For this review, use the dimensioned drawing (mm, ordinates from the lowest corner) and the shaded views. A direction names the side the tool comes from. Round coordinates to 2 decimals unless told otherwise and drop trailing zeros. Order: outer loops, then holes, each group sorted by start corner. A loop starts at its lowest first (then second) coordinate and runs counter-clockwise, first axis right, second up. Notation, with made-up numbers: (64, -14) - (121, -14) arc R34 ccw to (121, 21) - close; hole circle Ø3 at (-40, 89.25). An arc over 180 degrees is marked (long way). Use CSV: the item, a comma, the result in double quotes. Start each with the question number.
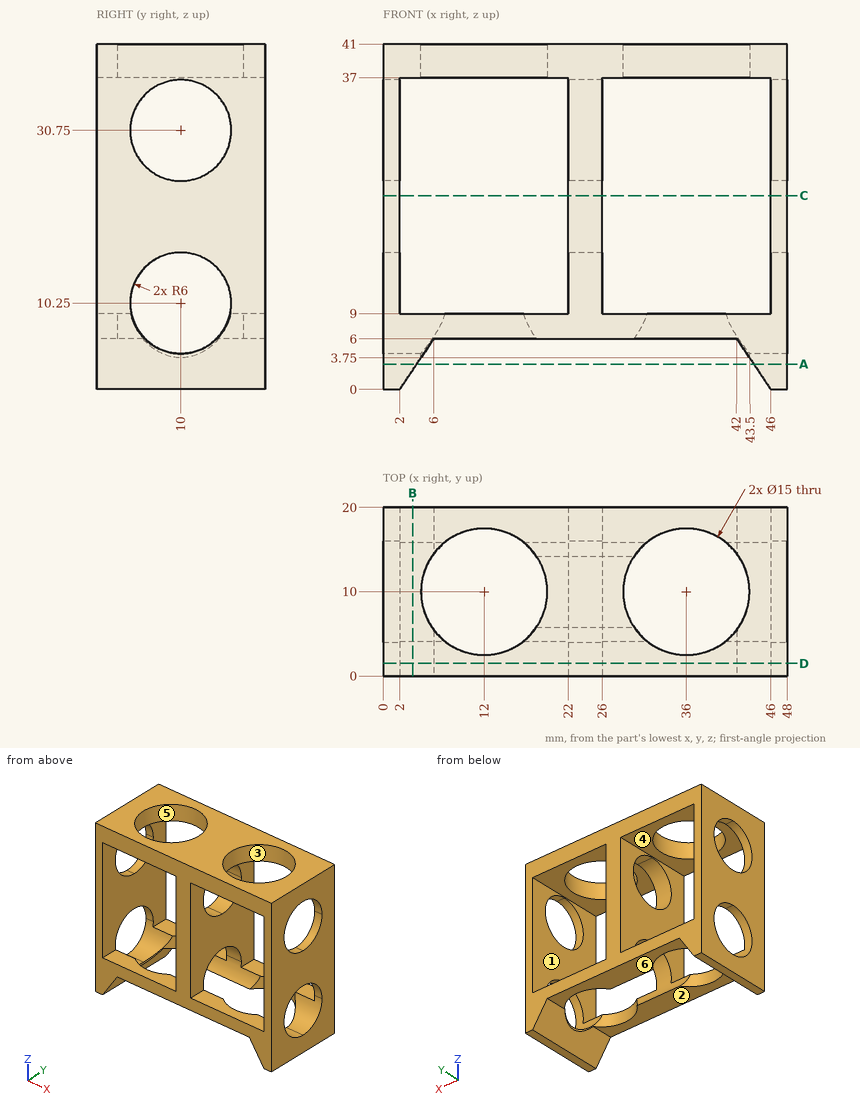
Q1. Take a section at D-D (y = 1.5). State the section outline as (x, z) points.
Q2. Take a section at B-B (x = 3.5). State the section outline as (y, z) points.
Q3. Take a section at C-C (z = 23). State the section outline as (x, y) points, plus the area to 3 significant figures.
Q4. Take a section at A-A (z = 3). State the section outline as (x, y) points, plus the area to 3 significant figures.
Q5. Clearance check with flat-ended pins moving along their axes: pin 1 (1.7 mm diameter, centred on x = 15, y = 3, fed in from -Z); pin 2 (1 mm diameter, centred on x = 25.5, y = 6.5, fed in from -Z); pin 3 (10 mm diameter, centred on x = 42, z = 25.5, fed in from -Y). State where each tip first meets the part, or that it passes through.
Q6. Tool access review of the marked faces 1, 2 and 3: name each direction out of +Z, -Z, +X, -X, +Y, -Y from which nothing blocks a thin tool from reaching the whole face with its end or side.
Q7. For L1, parallel to X at y = 12.25, z = 21; L2, parallel to Z at x = 12, y = 19; L3, parallel to X at y = 8.75, z = 39, list the stretches that pass through material, from the lowest coordinate up. Write a range as [from, to].
Q8. The part is to be moulded in two halves that separate along Z. For the marked faces 4, 5 and 6, say which applies: +Z half, -Z half, draft (parallel to the pull), parting line (faces both ways), or undercut.
Findings below:
1,outline,"(0, 0) - (2, 0) - (6, 6) - (42, 6) - (46, 0) - (48, 0) - (48, 41) - (0, 41) - close; hole (2, 9) - (22, 9) - (22, 37) - (2, 37) - close; hole (26, 9) - (46, 9) - (46, 37) - (26, 37) - close"
2,outline,"(0, 2.25) - (20, 2.25) - (20, 9) - (15.87, 9) arc R6 cw to (4.13, 9) - (0, 9) - close; (0, 37) - (20, 37) - (20, 41) - (0, 41) - close"
3,outline,"(0, 0) - (2, 0) - (2, 20) - (0, 20) - close; (22, 0) - (26, 0) - (26, 20) - (22, 20) - close; (46, 0) - (48, 0) - (48, 20) - (46, 20) - close"
3,area,"160 mm^2"
4,outline,"(0, 0) - (4, 0) - (4, 20) - (0, 20) - close; (44, 0) - (48, 0) - (48, 20) - (44, 20) - close"
4,area,"160 mm^2"
5,pin 1,"stops at z = 6"
5,pin 2,"stops at z = 14.72"
5,pin 3,"stops at y = 0"
6,face 1,"+Y, -Y"
6,face 2,"-Z, +Y, -Y"
6,face 3,"+Z, -Z"
7,L1,"x = [0, 2], [22, 26], [46, 48]"
7,L2,"z = [6, 9], [37, 41]"
7,L3,"x = [0, 4.6], [19.4, 28.6], [43.4, 48]"
8,face 4,"undercut"
8,face 5,"draft"
8,face 6,"-Z half"
